The model under review builds one solid part; all positions refer to its coordinate system, in mm. A direction names the side the tool comes from. Give positions to 0.01 mm unless a question says otherwise; leave off trailing zeros. Order: outer loops, then holes, each group sorted by start corner. A loop starts at its lowest first (then second) coordinate and runs counter-clockwise, first axis right, second up. Notation, with made-up numbers: (-16, 72) - (33, 72) arc R29 ccw to (33, 99) - close; hole circle Ø9 at (-17, 88.5). An arc over 180 degrees is marked (long way). Put each result on its own line as item: value.
```python
from build123d import *

# Parameters (mm, degrees)
SKETCH1_W           = 40
SKETCH1_H           = 20
BOSS_EXTRUDE1_DEPTH = 2
SKETCH2_W           = 14
SKETCH2_H           = 10
BOSS_EXTRUDE2_DEPTH = 11
SKETCH3_W           = 6.5
SKETCH3_H           = 13
BOSS_EXTRUDE3_DEPTH = 5


with BuildPart() as part:
    # Sketch1 → Boss-Extrude1 (new body)
    with BuildSketch(Plane(origin=(0, 0, 0), x_dir=(1, 0, 0), z_dir=(0, 1, 0))):
        Rectangle(SKETCH1_W, SKETCH1_H)
    extrude(amount=BOSS_EXTRUDE1_DEPTH)

    # Sketch2 → Boss-Extrude2 (add)
    with BuildSketch(Plane(origin=(0, 2, 0), x_dir=(1, 0, 0), z_dir=(0, 1, 0))):
        with Locations((13, 3)):
            Rectangle(SKETCH2_W, SKETCH2_H)
    extrude(amount=BOSS_EXTRUDE2_DEPTH)

    # Sketch3 → Boss-Extrude3 (add)
    with BuildSketch(Plane(origin=(0, 2, 0), x_dir=(1, 0, 0), z_dir=(0, 1, 0))):
        with Locations((-16.25, 3.5)):
            Rectangle(SKETCH3_W, SKETCH3_H)
    extrude(amount=BOSS_EXTRUDE3_DEPTH)


solid = part.part
```
(1) Take a section at C-C, the plane z = -8.5. Write out the cut boundary in (x, y), then the cut area to 4 significant figures.
The answers:
outline: (-20, 0) - (20, 0) - (20, 2) - (-13, 2) - (-13, 7) - (-19.5, 7) - (-19.5, 2) - (-20, 2) - close
area: 112.5 mm^2
(2) The part is to be moulded in two halves that separate along X. For faces 1 (the flat face through (20, 6, -2)), 2 (the flat face through (0, 0, 0)), 3 (the flat face through (6, 7, -3)), say which applies: pulls with the +X half, pulls with the -X half, needs draft (parallel to the pull), parting line crosses it, or undercut.
The answers:
face 1: pulls with the +X half
face 2: needs draft
face 3: undercut
(3) Take a section at D-D, the plane y = 8.75. Write out the cut boundary in (x, z).
The answers:
outline: (6, -8) - (20, -8) - (20, 2) - (6, 2) - close
(4) Clearance check with flat-ended pins moving along their axes: pin 1 Ø3 at (x, z) = (-16.5, -0.5) entering from +Y; pin 2 Ø4 at (y, z) = (5.5, -6) entering from -X; pin 3 Ø1.5 at (x, y) = (-15, 5) entering from +Z. State where each tip first meets the part, or that it passes through.
The answers:
pin 1: y = 7
pin 2: x = -19.5
pin 3: z = 3
(5) Take a section at B-B, the plane x = 17. Write out the cut boundary in (y, z), then the cut area to 3 significant figures.
The answers:
outline: (0, -10) - (2, -10) - (2, -8) - (13, -8) - (13, 2) - (2, 2) - (2, 10) - (0, 10) - close
area: 150 mm^2
(6) Wall thickness on L1, parallel to X at y = 6.5, z = -5; L2, parallel to Y at x = -5.5, z = -0.5; L3, parallel to Z at x = 7, y = 4.5: over which ranges is each line inside the solid? List them lowest first.
The answers:
L1: -19.5 to -13, 6 to 20
L2: 0 to 2
L3: -8 to 2
(7) For faces 4 (the flat face through (13, 7, 2)), 5 (the flat face through (-13, 4, -3)), 6 (the flat face through (-19.5, 4, -3)), 7 (the flat face through (-16, 4, 3)), list the 3-axis set-ups (+Z, -Z, +X, -X, +Y, -Y) from which the entire face can be reached by the end or side of a thin tool; tool diameter is ignored.
The answers:
face 4: +Z, +X, +Y
face 5: +Z, -Z, +Y
face 6: +Z, -Z, -X, +Y
face 7: +Z, +X, -X, +Y
(8) Take a section at A-A, the plane y = 5.75. Write out the cut boundary in (x, z).
The answers:
outline: (-19.5, -10) - (-13, -10) - (-13, 3) - (-19.5, 3) - close; (6, -8) - (20, -8) - (20, 2) - (6, 2) - close
